Solid Edge part; units mm, degrees
sketch "Sketch1" plane through (0, 0, 0) normal (0, 0, 1) x (1, 0, 0)
  circle A0 centre (0, 0) radius 12.7
extrude "Protrusion1" add sketch "Sketch1" along normal blind 254
sketch "Sketch2" plane through (0, 0, 254) normal (0, 0, 1) x (1, 0, 0)
  circle A0 centre (0, 0) radius 19.05
extrude "ExtrudedProtrusion_2" add sketch "Sketch2" against normal blind 203.2
sketch "Sketch3" plane through (0, 0, 0) normal (0, 0, -1) x (-1, 0, 0)
  line L0 (-2.9642, 14.7392) -> (2.9642, 14.7392)
  line L1 (2.9642, 14.7392) -> (2.9642, 10.6608)
  line L2 (2.9642, 10.6608) -> (-2.9642, 10.6608)
  line L3 (-2.9642, 10.6608) -> (-2.9642, 14.7392)
extrude "ExtrudedCutout_1" cut sketch "Sketch3" against normal blind 50.8
sketch "Sketch4" plane through (0, 0, 50.8) normal (0, 0, -1) x (-1, 0, 0)
  line L0 (-4.8624, 22.4209) -> (4.8624, 22.4209)
  line L1 (4.8624, 22.4209) -> (4.8624, 15.6791)
  line L2 (4.8624, 15.6791) -> (-4.8624, 15.6791)
  line L3 (-4.8624, 15.6791) -> (-4.8624, 22.4209)
extrude "ExtrudedCutout_2" cut sketch "Sketch4" against normal blind 224.5097
sketch "Sketch5" plane through (0, -0.3155, 50.8) normal (0, 0, -1) x (1, 0, 0)
  circle A0 centre (0, -0.3155) radius 31.75
extrude "ExtrudedProtrusion_3" add sketch "Sketch5" along normal blind 6.35
chamfer "Chamfer_1" distance 1.27 angle 45 1 edges at (-31.75, 0, 44.45)
hole "Hole_1" at (0, 0, 254) direction (0, 0, -1) diameter 4.9759 depth 76.2 counterbore diameter 9.9212 counterbore depth 5.588 thread major 6.35 thread length 50.8
sketch "Sketch6" plane through (0, 0, 0) normal (0, 0, 1) x (1, 0, 0)
  circle A0 centre (0, 0) radius 12.7
extrude "ExtrudedCutout_3" cut sketch "Sketch6" along normal blind 12.7
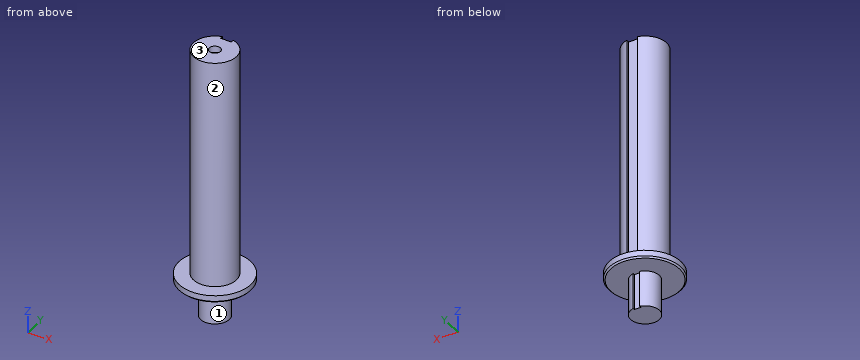
Here's how the part is built. I have some questions about the finished solid (model axes, mm). Face numbers are marked on the shaded views. A direction names the side the tool comes from. Coordinates: 2 decimals unless noted, no trailing zeros. Write each loop counter-clockwise with the first axis right and the second up, starting at its lowest first coordinate (ties: lowest second). Pieces come first, ordered by that corner, then holes. Notation, with made-up numbers: (52.25, -15.5) - (65.25, -15.5) arc R21 cw to (65.25, 8.5) - close; hole circle Ø10 at (64.25, -13). An arc over 180 degrees is marked (long way). One line per item, written item: value.
1) Suppose I cut it at A-A on z = 212.5. Write out the boundary of the cut face in (x, y).
Model answer:
outline: (-4.86, 15.68) - (-4.86, 18.42) arc R19.05 ccw (long way) to (4.86, 18.42) - (4.86, 15.68) - close; hole circle Ø4.98 at (0, 0)
2) Suppose I cut it at B-B on y = 0. Write out the boundary of the cut face in (x, z), and give its area (3 significant figures).
Model answer:
outline: (-31.75, 45.72) - (-30.48, 44.45) - (-12.7, 44.45) - (-12.7, 12.7) - (12.7, 12.7) - (12.7, 44.45) - (30.48, 44.45) - (31.75, 45.72) - (31.75, 50.8) - (19.05, 50.8) - (19.05, 254) - (4.96, 254) - (4.96, 248.41) - (2.49, 248.41) - (2.49, 177.8) - (-2.49, 177.8) - (-2.49, 248.41) - (-4.96, 248.41) - (-4.96, 254) - (-19.05, 254) - (-19.05, 50.8) - (-31.75, 50.8) - close
area: 8,540 mm²
3) I need wall thicknesses on line 1 along Y through (x, z) = (0, 209); line 2 along Y through (x, z) = (0, 249); line 3 along X through (y, z) = (0, 250). Which ranges of each line are inside material? Lowest first, please.
Model answer:
line 1: y = -19.05 to -2.49, 2.49 to 15.68
line 2: y = -19.05 to -4.96, 4.96 to 15.68
line 3: x = -19.05 to -4.96, 4.96 to 19.05
4) I'm going to push flat-ended pins straight in: P1, Ø0.8, axis at y = 11.5, z = 25, coming from the +X side; P2, Ø3, axis at y = 2, z = 136, coming from the +X side; P3, Ø1.4, axis at y = 11.5, z = 25.5, coming from the -X side. Where does each tip first touch, or does it pass through?
Model answer:
P1: stops at x = 6.17
P2: stops at x = 19.04
P3: stops at x = -6.68
5) Suppose I cut it at C-C on x = 0. Write out the boundary of the cut face in (y, z), and give its area (3 significant figures).
Model answer:
outline: (-31.75, 45.72) - (-30.48, 44.45) - (-12.7, 44.45) - (-12.7, 12.7) - (10.66, 12.7) - (10.66, 44.45) - (30.48, 44.45) - (31.75, 45.72) - (31.75, 50.8) - (15.68, 50.8) - (15.68, 254) - (4.96, 254) - (4.96, 248.41) - (2.49, 248.41) - (2.49, 177.8) - (-2.49, 177.8) - (-2.49, 248.41) - (-4.96, 248.41) - (-4.96, 254) - (-19.05, 254) - (-19.05, 50.8) - (-31.75, 50.8) - close
area: 7,790 mm²
6) Suppose I cut it at D-D on z = 140.5. Write out the boundary of the cut face in (x, y), and give its area (3 significant figures).
Model answer:
outline: (-4.86, 15.68) - (-4.86, 18.42) arc R19.05 ccw (long way) to (4.86, 18.42) - (4.86, 15.68) - close
area: 1,110 mm²
7) On a 3-axis mill with a long thin cutter (end or side, diameter ignored), from which of +Z, -Z, +X, -X, +Y, -Y can I reach the whole of each face in a straight line? I mean the marked faces 1, 2 and 3. Say none if no direction works.
Model answer:
face 1: -Z
face 2: +Z
face 3: +Z, +X, -X, +Y, -Y
